```python
from build123d import *

# Parameters (mm, degrees)
SKETCH_W         = 76.2
SKETCH_H         = 431.8
PAD_DEPTH        = 6.35
HOLE_D           = 7.1
HOLE_CSINK_D     = 13.49375
HOLE_CSINK_ANGLE = 81


with BuildPart() as part:
    # Sketch → Pad (new body)
    with BuildSketch(Plane.XY):
        Rectangle(SKETCH_W, SKETCH_H)
    extrude(amount=PAD_DEPTH)

    # Hole (through all)
    with Locations(Plane.XY.offset(6.35)):
        with Locations((-25.4, 190.5), (-25.4, 0), (-25.4, 107.95), (-25.4, -190.5), (-25.4, -107.95), (25.4, -190.5), (25.4, -107.95), (25.4, 0), (25.4, 107.95), (25.4, 190.5)):
            CounterSinkHole(HOLE_D / 2, HOLE_CSINK_D / 2, counter_sink_angle=HOLE_CSINK_ANGLE)


solid = part.part
```
Design review of the part built by this model. Coordinates are the model's own, in mm. Coordinates: 2 decimals unless noted, no trailing zeros. Loops run counter-clockwise (first coordinate to the right, second up) from the corner with the lowest first, then second, coordinate; pieces in that order, holes last.
Q1. We need section A-A on y = 190.5. State the section outline as (x, z) points.
Reported:
outline: (-38.1, 0) - (-28.95, 0) - (-28.95, 2.61) - (-32.15, 6.35) - (-38.1, 6.35) - close; (-21.85, 0) - (21.85, 0) - (21.85, 2.61) - (18.65, 6.35) - (-18.65, 6.35) - (-21.85, 2.61) - close; (28.95, 0) - (38.1, 0) - (38.1, 6.35) - (32.15, 6.35) - (28.95, 2.61) - close
Q2. The part is to be moulded in two halves that separate along X. For faces 1 (the face through (-28.934, -106.837, 2.789)), 2 (the face through (-1, 3, 0)), say which applies: +X half, -X half, draft (parallel to the pull), parting line (faces both ways), or undercut.
Reported:
face 1: undercut
face 2: draft
Q3. To check wall thickness, follow line 1 (Y direction, x = 25.4, z = 1.9); line 2 (X direction, y = 107.95, z = 0.8); line 3 (X direction, y = 104.5, z = 3.5). State the ranges of each line that lie inside material, in increasing order.
Reported:
line 1: y = -215.9 to -194.05, -186.95 to -111.5, -104.4 to -3.55, 3.55 to 104.4, 111.5 to 186.95, 194.05 to 215.9
line 2: x = -38.1 to -28.95, -21.85 to 21.85, 28.95 to 38.1
line 3: x = -38.1 to -27.99, -22.81 to 22.81, 27.99 to 38.1
Q4. We need section B-B on z = 4.5. State how many separate pieces and enclosed holes the cut face has, and give its area (3 significant figures).
Reported:
separate pieces: 1
enclosed holes: 10
area: 32,100 mm2
Q5. For pin 1 (9 mm diameter, centred on x = -25.4, y = 0, fed in from +Z), flat-tipped, find the tip position at first contact; note if it passes through.
Reported:
pin 1: stops at z = 3.72
